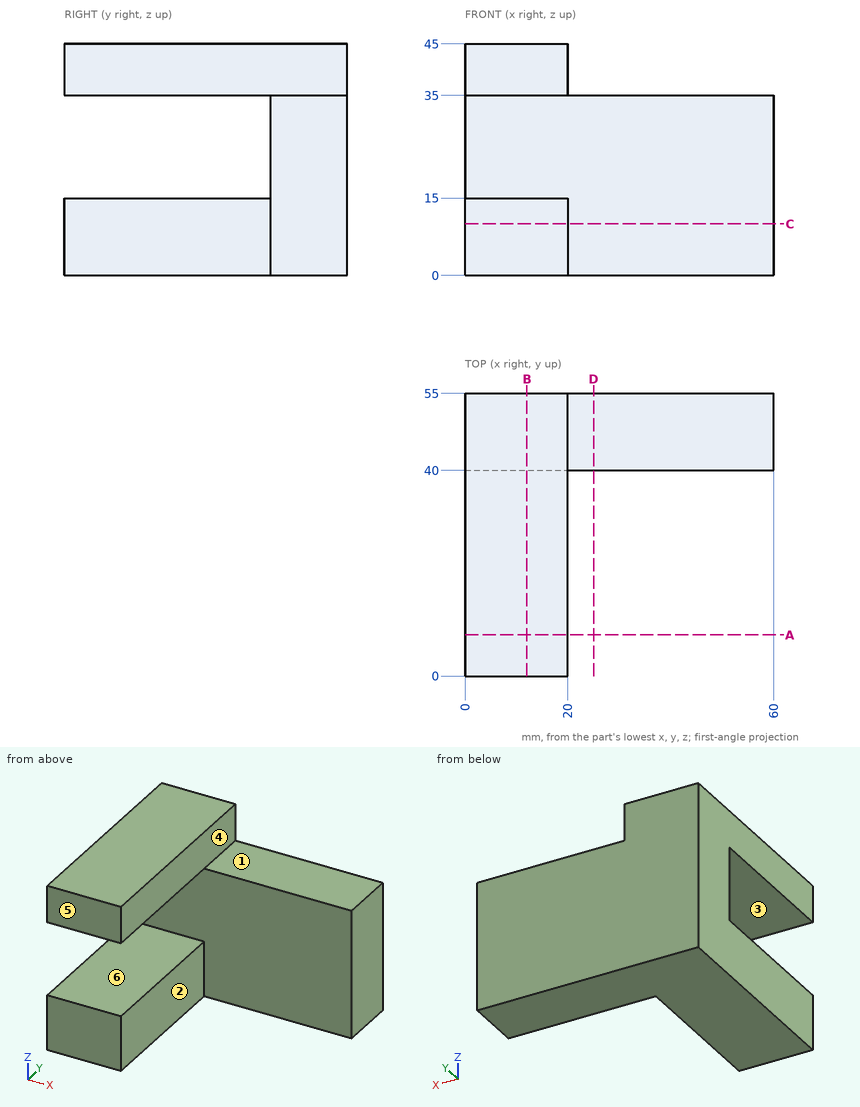
The figure shows three views and two pictorial views of one solid part (mm, origin at its lowest corner). Answer the questions. A direction names the side the tool comes from. Round coordinates to 2 decimals unless told otherwise and drop trailing zeros. Write each loop counter-clockwise with the first axis right and the second up, starting at its lowest first coordinate (ties: lowest second). Pieces come first, ordered by that corner, then holes. Notation, with made-up numbers: (-26.5, -16.75) -> (12.5, -16.75) arc R18 cw to (12.5, 13.25) -> close; hole circle Ø7 at (58.25, 35.25). An arc over 180 degrees is marked (long way). Answer as a JSON object with one key per item and string values. Group by question number.
Q1. Section A-A (y = 8) is taken. Write down the section's boundary in (x, z).
Q2. Section C-C (z = 10) is taken. Write down the section's boundary in (x, y), plus the area to 3 significant figures.
Q3. Section B-B (x = 12) is taken. Write down the section's boundary in (y, z).
Q4. Each of these flat-tipped pins is pushed along its axis until it touches: pin 1 Ø16.5 at (y, z) = (23.5, 6.5) entering from +X; pin 2 Ø8 at (y, z) = (13.5, 29) entering from -X; pin 3 Ø7.5 at (x, y) = (47.5, 46.5) entering from +Z. Where does it stop, or does it pass through?
Q5. Section D-D (x = 25) is taken. Write down the section's boundary in (y, z), plus the area to 3 significant figures.
Q6. Which of the six approach directions +Z, -Z, +X, -X, +Y, -Y give full straight-line access (tool end or side, diameter ignored) to the marked faces 4, 5 and 6?
Q7. Straight lines are drawn through the part: line 1 along Z through (x, y) = (18.5, 32.5); line 2 along Y through (x, z) = (50, 5); line 3 along Z through (x, y) = (47, 48.5). For each, find the intervals that lie inside material, in ascending order.
Q8. Determine the mould class of the marked faces 1, 2 and 3 for opening direction Z: pulls with the +Z half, pulls with the -Z half, needs draft (parallel to the pull), parting line crosses it, or undercut.
Check values:
{
 "1": {"outline": "(0, 0) -> (20, 0) -> (20, 15) -> (0, 15) -> close; (0, 35) -> (20, 35) -> (20, 45) -> (0, 45) -> close"},
 "2": {"outline": "(0, 0) -> (20, 0) -> (20, 40) -> (60, 40) -> (60, 55) -> (0, 55) -> close", "area": "1,700 mm^2"},
 "3": {"outline": "(0, 0) -> (55, 0) -> (55, 45) -> (0, 45) -> (0, 35) -> (40, 35) -> (40, 15) -> (0, 15) -> close"},
 "4": {"pin 1": "x = 20", "pin 2": "through", "pin 3": "z = 35"},
 "5": {"outline": "(40, 0) -> (55, 0) -> (55, 35) -> (40, 35) -> close", "area": "525 mm^2"},
 "6": {"face 4": "+Z, +X, +Y, -Y", "face 5": "+Z, -Z, +X, -X, -Y", "face 6": "+X, -X, -Y"},
 "7": {"line 1": "0 to 15, 35 to 45", "line 2": "40 to 55", "line 3": "0 to 35"},
 "8": {"face 1": "pulls with the +Z half", "face 2": "needs draft", "face 3": "undercut"}
}
